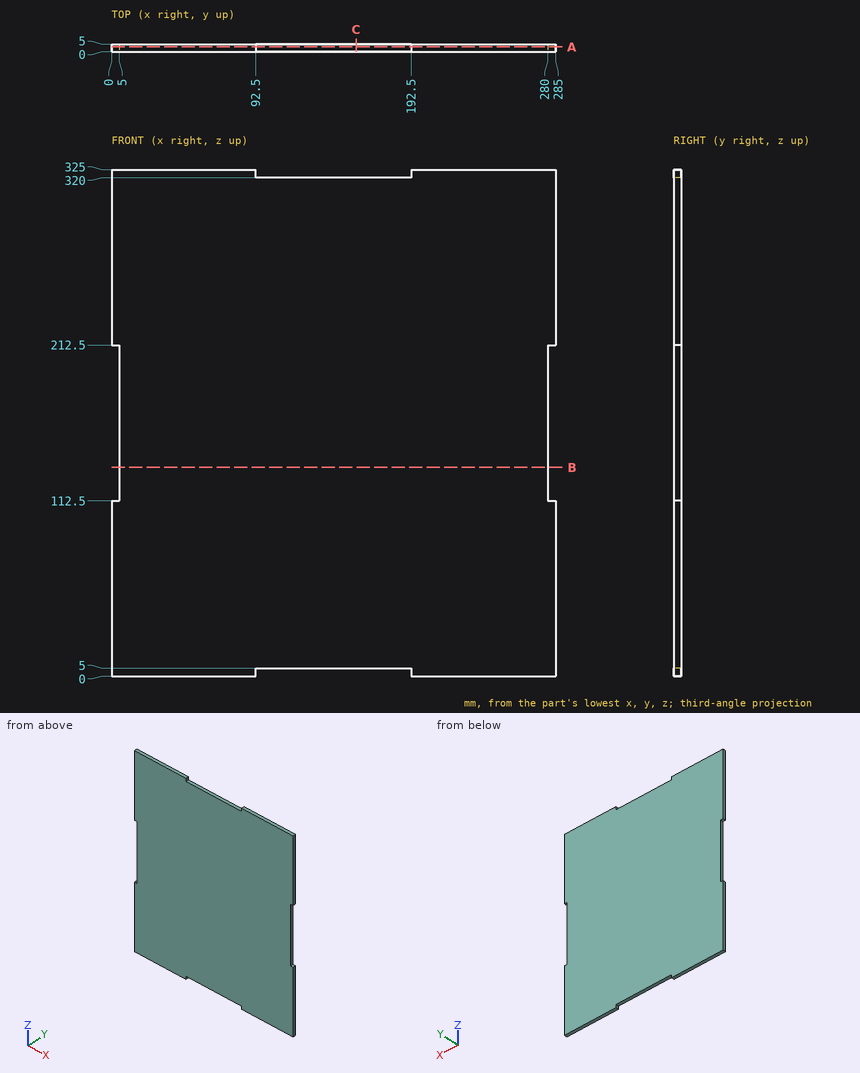
Print and shaded views of the part. All mm, measured from the part's lowest x, y and z. Give positions to 0.01 mm unless a question says otherwise; leave off trailing zeros. Write each loop counter-clockwise with the first axis right and the second up, starting at its lowest first coordinate (ties: lowest second). Pieces come first, ordered by that corner, then holes. Notation, with made-up numbers: (54.25, -4.75) -> (61.25, -4.75) arc R15 cw to (61.25, 12.25) -> close; hole circle Ø11 at (9.5, -30). An arc over 180 degrees is marked (long way). Use CSV: the item, a comma, the result in double quotes. Start each with the question number.
1) Pin check, flat tips, straight feed: P1, Ø1.5, axis at x = 157, y = 2.5, coming from the -Z side; P2, Ø2.5, axis at y = 3.5, z = 184.5, coming from the +X side. Stop position of each tip, or through.
2) Drill centre lines: L1, parallel to Z at x = 153, y = 0.7; L2, parallel to X at y = 3.95, z = 182.5. Where is each one in solid material? Low to high.
3) Cut at A-A on y = 3.2. List the corners of the cut face in (x, z).
4) Cut at B-B on z = 134. List the corners of the cut face in (x, y).
5) Cut at C-C on x = 157. List the corners of the cut face in (y, z), plus the area to 4 significant figures.
Final values:
1,P1,"stops at z = 5"
1,P2,"stops at x = 280"
2,L1,"z = 5 to 320"
2,L2,"x = 5 to 280"
3,outline,"(0, 0) -> (92.5, 0) -> (92.5, 5) -> (192.5, 5) -> (192.5, 0) -> (285, 0) -> (285, 112.5) -> (280, 112.5) -> (280, 212.5) -> (285, 212.5) -> (285, 325) -> (192.5, 325) -> (192.5, 320) -> (92.5, 320) -> (92.5, 325) -> (0, 325) -> (0, 212.5) -> (5, 212.5) -> (5, 112.5) -> (0, 112.5) -> close"
4,outline,"(5, 0) -> (280, 0) -> (280, 5) -> (5, 5) -> close"
5,outline,"(0, 5) -> (5, 5) -> (5, 320) -> (0, 320) -> close"
5,area,"1,575 mm2"
